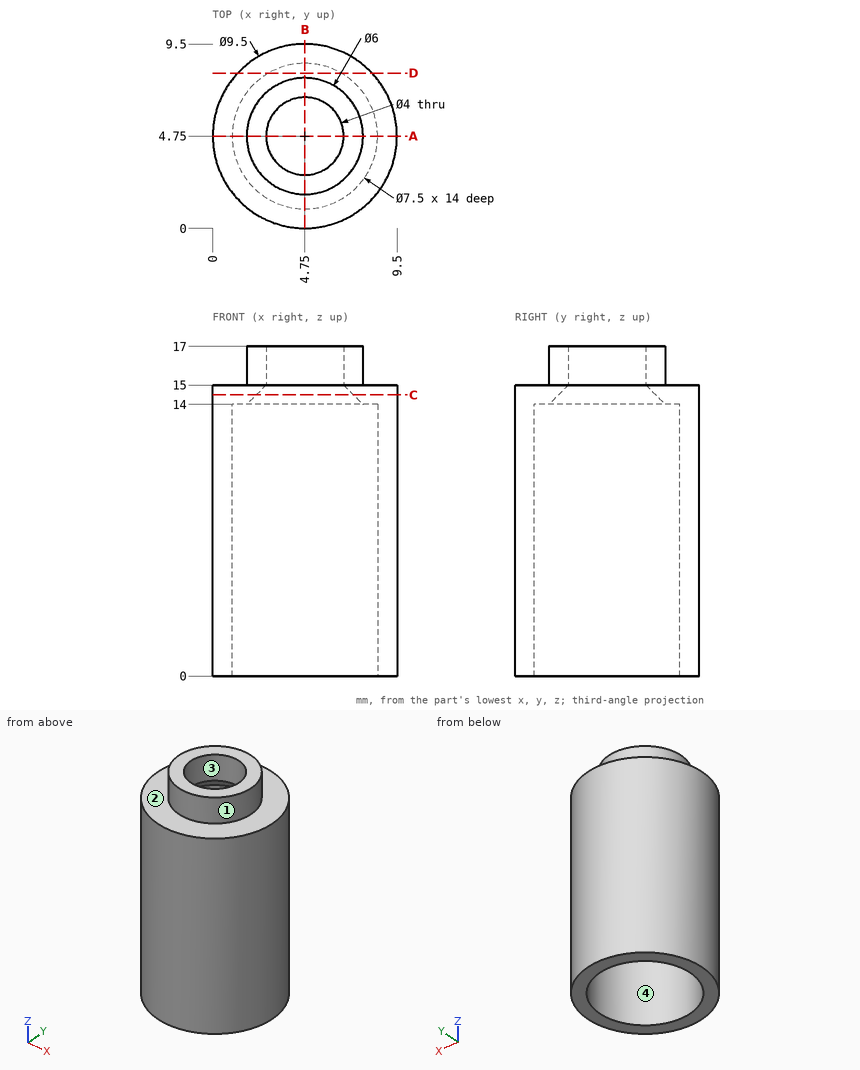
Can you work these out from the drawing? Everything is in mm from the part's minimum corner. Coordinates: 2 decimals unless noted, no trailing zeros. Loops run counter-clockwise (first coordinate to the right, second up) from the corner with the lowest first, then second, coordinate; pieces in that order, holes last.
1) For pin 1 (2 mm diameter, centred on y = 1.5, z = 2.5, fed in from -X); pin 2 (5 mm diameter, centred on x = 4.75, y = 4.75, fed in from -Z); pin 3 (1.5 mm diameter, centred on y = 2, z = 10.5, fed in from +X), each with a flat end and sliding along its axis, tell me the tip position at first contact or that it passes through.
2) Thinking about a two-plate mould opening in X: for the marked faces 1, 2, 3 and 4, which applies, pulls with the +X half, pulls with the -X half, needs draft (parallel to the pull), parting line crosses it, or undercut?
3) Imagine slicing it at D-D on y = 8. List the corners of the cut face in (x, z) for me, plus the area to 3 significant figures.
4) Imagine slicing it at C-C on z = 14.5. List the corners of the cut face in (x, y) for me.
5) I need wall thicknesses on probe 1 along Y at (x, z) = (4.75, 16.15); probe 2 along Y at (x, z) = (4.75, 9.5); probe 3 along X at (y, z) = (1.75, 5.25). Which ranges of each line are inside material? Lowest first, please.
6) Imagine slicing it at A-A on y = 4.75. List the corners of the cut face in (x, z) for me, plus the area to 3 significant figures.
Completed:
1. pin 1: stops at x = 0.57
1. pin 2: stops at z = 14.5
1. pin 3: stops at x = 9.06
2. face 1: parting line crosses it
2. face 2: needs draft
2. face 3: undercut
2. face 4: undercut
3. outline: (1.29, 0) - (2.88, 0) - (2.88, 14) - (6.62, 14) - (6.62, 0) - (8.21, 0) - (8.21, 15) - (1.29, 15) - close
3. area: 51.5 mm2
4. outline: circle Ø9.5 at (4.75, 4.75); hole circle Ø5 at (4.75, 4.75)
5. probe 1: y = 1.75 to 2.75, 6.75 to 7.75
5. probe 2: y = 0 to 1, 8.5 to 9.5
5. probe 3: x = 1.07 to 2.5, 7 to 8.43
6. outline: (0, 0) - (1, 0) - (1, 14) - (1.75, 14) - (2.75, 15) - (2.75, 17) - (1.75, 17) - (1.75, 15) - (0, 15) - close; (6.75, 15) - (7.75, 14) - (8.5, 14) - (8.5, 0) - (9.5, 0) - (9.5, 15) - (7.75, 15) - (7.75, 17) - (6.75, 17) - close
6. area: 36.5 mm2
